Drawing for the job (mm, zero at the part's lowest x, y, z). A direction names the side the tool comes from. Give positions to 0.01 mm unless a question says otherwise; leave off trailing zeros. Write each loop counter-clockwise with the first axis right and the second up, starting at its lowest first coordinate (ties: lowest second). Pieces come first, ordered by that corner, then holes.
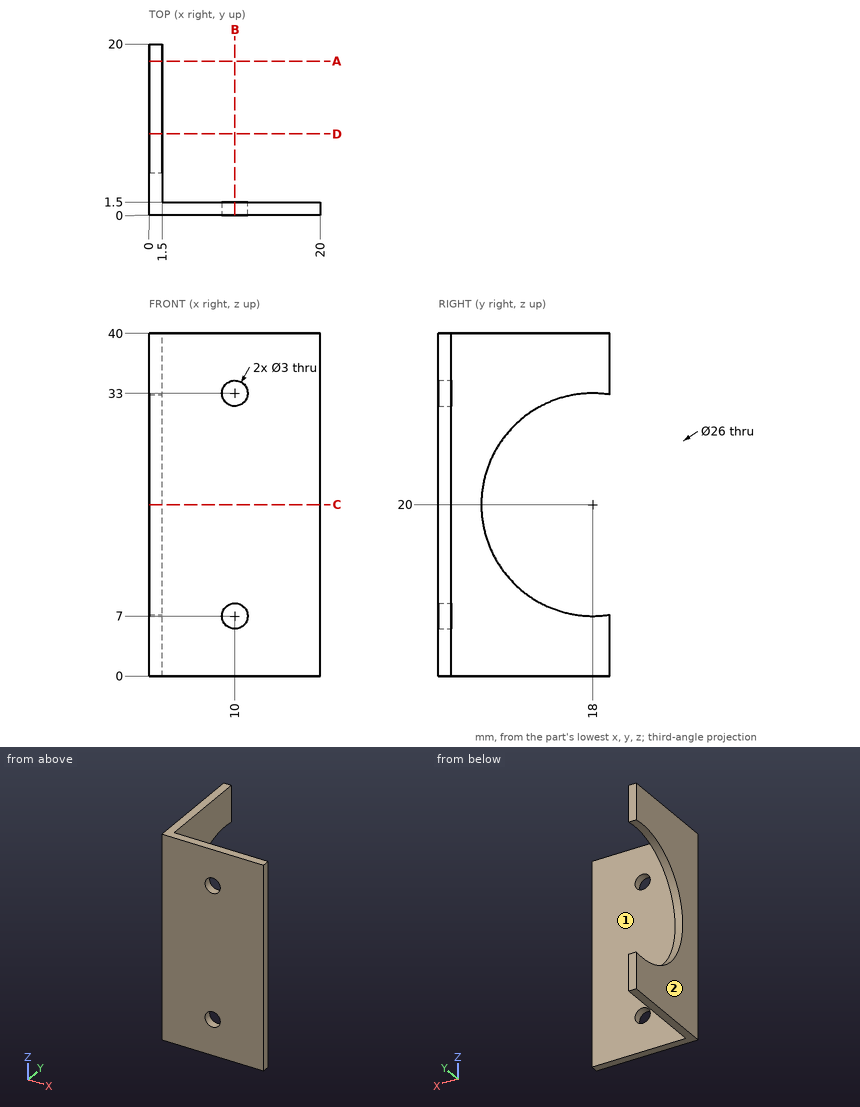
1. Slice it at A-A, the plane y = 18. Write the cut outline in (x, z).
Calculated:
outline: (0, 0) - (1.5, 0) - (1.5, 7) - (0, 7) - close; (0, 33) - (1.5, 33) - (1.5, 40) - (0, 40) - close
2. Pin check, flat tips, straight feed: P1, Ø3.5, axis at x = 10, z = 33, coming from the +Y side; P2, Ø8, axis at x = 8.5, y = 15.5, coming from the +Z side (3 decimals). Stop position of each tip, or through.
Calculated:
P1: stops at y = 1.5
P2: passes through
3. Probe probe 1 along Z at (x, y) = (10, 1.05); probe 2 along Z at (x, y) = (0.7, 18); probe 3 along X at (y, z) = (5.5, 31.5). List the from-to ranges inside material, lowest first.
Calculated:
probe 1: z = 0 to 5.5, 8.5 to 31.5, 34.5 to 40
probe 2: z = 0 to 7, 33 to 40
probe 3: x = 0 to 1.5
4. Slice it at B-B, the plane x = 10. Write the cut outline in (y, z).
Calculated:
outline: (0, 0) - (1.5, 0) - (1.5, 5.5) - (0, 5.5) - close; (0, 8.5) - (1.5, 8.5) - (1.5, 31.5) - (0, 31.5) - close; (0, 34.5) - (1.5, 34.5) - (1.5, 40) - (0, 40) - close
5. Which spindle directions (+Z, -Z, +X, -X, +Y, -Y) get a long thin tool onto all of the face, cutting with end or side? Do the marked faces 1 and 2. Say none if no direction does.
Calculated:
face 1: +Z, -Z, +X, +Y
face 2: +Z, -Z, -X, +Y, -Y
6. Slice it at C-C, the plane z = 20. Write the cut outline in (x, y).
Calculated:
outline: (0, 0) - (20, 0) - (20, 1.5) - (1.5, 1.5) - (1.5, 5) - (0, 5) - close
7. Slice it at D-D, the plane y = 9.5. Write the cut outline in (x, z).
Calculated:
outline: (0, 0) - (1.5, 0) - (1.5, 10.16) - (0, 10.16) - close; (0, 29.84) - (1.5, 29.84) - (1.5, 40) - (0, 40) - close
